from build123d import *

# Parameters (mm, degrees)
SKETCH1_W           = 914.4
SKETCH1_H           = 609.6
BOSS_EXTRUDE1_DEPTH = 6.35
SKETCH2_W           = 571.5
SKETCH2_H           = 266.7
CUT_EXTRUDE1_DEPTH  = 7.35
SKETCH3_W           = 101.6
SKETCH3_H           = 50.8
CUT_EXTRUDE2_DEPTH  = 7.35
FILLET1_R           = 12.7
SKETCH4_R           = 3.175
CUT_EXTRUDE3_DEPTH  = 7.35
SKETCH6_R           = 3.302
CUT_EXTRUDE5_DEPTH  = 6.35


with BuildPart() as part:
    # Sketch1 → Boss-Extrude1 (new body)
    with BuildSketch(Plane.ZY.offset(304.8)):
        with Locations((0, 304.8)):
            Rectangle(SKETCH1_W, SKETCH1_H)
    extrude(amount=BOSS_EXTRUDE1_DEPTH)

    # Sketch2 → Cut-Extrude1 (cut, through all)
    with BuildSketch(Plane.ZY.offset(311.15)):
        with Locations((0, 330.2)):
            Rectangle(SKETCH2_W, SKETCH2_H)
    extrude(amount=-CUT_EXTRUDE1_DEPTH, mode=Mode.SUBTRACT)

    # Sketch3 → Cut-Extrude2 (cut, through all)
    with BuildSketch(Plane.ZY.offset(311.15)):
        with Locations((-330.2, 69.85)):
            Rectangle(SKETCH3_W, SKETCH3_H)
        with Locations((330.2, 69.85)):
            Rectangle(SKETCH3_W, SKETCH3_H)
    extrude(amount=-CUT_EXTRUDE2_DEPTH, mode=Mode.SUBTRACT)

    # Fillet1
    fillet1_edges = [part.edges().sort_by_distance(p)[0] for p in [
        (-307.975, 196.85, -285.75),
        (-307.975, 463.55, -285.75),
        (-307.975, 463.55, 285.75),
        (-307.975, 196.85, 285.75),
        (-307.975, 44.45, -381),
        (-307.975, 95.25, -381),
        (-307.975, 95.25, -279.4),
        (-307.975, 44.45, -279.4),
        (-307.975, 95.25, 279.4),
        (-307.975, 95.25, 381),
        (-307.975, 44.45, 381),
        (-307.975, 44.45, 279.4),
    ]]
    fillet(fillet1_edges, radius=FILLET1_R)

    # Sketch4 → Cut-Extrude3 (cut, through all)
    with BuildSketch(Plane.ZY.offset(311.15)):
        with Locations((323.85, 244.475)):
            Circle(SKETCH4_R)
        with Locations((-323.85, 244.475)):
            Circle(SKETCH4_R)
        with Locations((-107.95, 158.75)):
            Circle(SKETCH4_R)
        with Locations((0, 158.75)):
            Circle(SKETCH4_R)
        with Locations((215.9, 158.75)):
            Circle(SKETCH4_R)
        with Locations((323.85, 158.75)):
            Circle(SKETCH4_R)
        with Locations((-323.85, 158.75)):
            Circle(SKETCH4_R)
        with Locations((-215.9, 158.75)):
            Circle(SKETCH4_R)
        with Locations((266.7, 31.75)):
            Circle(SKETCH4_R)
        with Locations((393.7, 31.75)):
            Circle(SKETCH4_R)
        with Locations((266.7, 107.95)):
            Circle(SKETCH4_R)
        with Locations((393.7, 107.95)):
            Circle(SKETCH4_R)
        with Locations((-266.7, 31.75)):
            Circle(SKETCH4_R)
        with Locations((-393.7, 31.75)):
            Circle(SKETCH4_R)
        with Locations((-393.7, 107.95)):
            Circle(SKETCH4_R)
        with Locations((-266.7, 107.95)):
            Circle(SKETCH4_R)
        with Locations((323.85, 330.2)):
            Circle(SKETCH4_R)
        with Locations((323.85, 415.925)):
            Circle(SKETCH4_R)
        with Locations((323.85, 501.65)):
            Circle(SKETCH4_R)
        with Locations((215.9, 501.65)):
            Circle(SKETCH4_R)
        with Locations((107.95, 501.65)):
            Circle(SKETCH4_R)
        with Locations((0, 501.65)):
            Circle(SKETCH4_R)
        with Locations((-107.95, 501.65)):
            Circle(SKETCH4_R)
        with Locations((-215.9, 501.65)):
            Circle(SKETCH4_R)
        with Locations((-323.85, 501.65)):
            Circle(SKETCH4_R)
        with Locations((-323.85, 415.925)):
            Circle(SKETCH4_R)
        with Locations((-323.85, 330.2)):
            Circle(SKETCH4_R)
    extrude(amount=-CUT_EXTRUDE3_DEPTH, mode=Mode.SUBTRACT)

    # Sketch6 → Cut-Extrude5 (cut)
    with BuildSketch(Plane.ZY.offset(311.15)):
        with Locations((431.8, 164.084)):
            Circle(SKETCH6_R)
        with Locations((431.8, 230.124)):
            Circle(SKETCH6_R)
        with Locations((431.8, 296.164)):
            Circle(SKETCH6_R)
        with Locations((431.8, 362.204)):
            Circle(SKETCH6_R)
        with Locations((431.8, 428.244)):
            Circle(SKETCH6_R)
        with Locations((431.8, 494.284)):
            Circle(SKETCH6_R)
        with Locations((-431.8, 230.124)):
            Circle(SKETCH6_R)
        with Locations((-431.8, 296.164)):
            Circle(SKETCH6_R)
        with Locations((-431.8, 362.204)):
            Circle(SKETCH6_R)
        with Locations((-431.8, 428.244)):
            Circle(SKETCH6_R)
        with Locations((-431.8, 494.284)):
            Circle(SKETCH6_R)
        with Locations((-431.8, 164.084)):
            Circle(SKETCH6_R)
    extrude(amount=-CUT_EXTRUDE5_DEPTH, mode=Mode.SUBTRACT)


solid = part.part
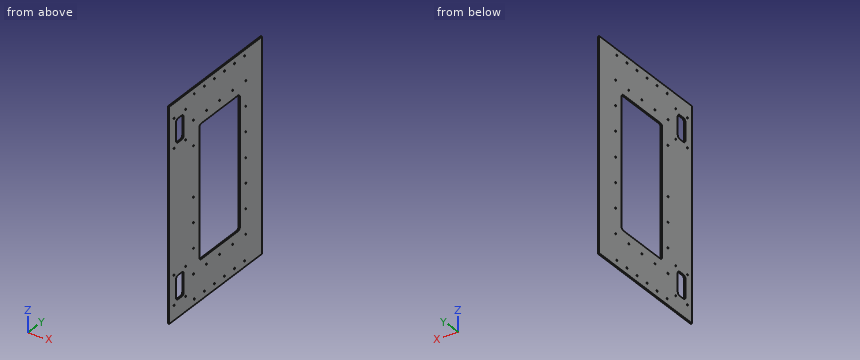
Model file for the job. Use its own axes, mm. Give positions to 0.01 mm unless a question says otherwise; leave off trailing zeros. Order: outer loops, then holes, each group sorted by start corner. A loop starts at its lowest first (then second) coordinate and runs counter-clockwise, first axis right, second up. Notation, with made-up numbers: (16, 59) -> (38, 59) arc R20 cw to (38, 81) -> close; hole circle Ø3 at (30.25, 13). An arc over 180 degrees is marked (long way). Use CSV: the item, a comma, the result in double quotes.
1. Band-saw the part on A-A, the plane z = 182. Give the cut face in (x, y).
Outcome:
outline,"(-311.15, 0) -> (-304.8, 0) -> (-304.8, 196.85) -> (-311.15, 196.85) -> close; (-311.15, 463.55) -> (-304.8, 463.55) -> (-304.8, 609.6) -> (-311.15, 609.6) -> close"
2. Drill centre lines: line 1 along Y through (x, z) = (-308.25, 215.9) (3 decimals); line 2 along Z through (x, y) = (-307.5, 301); line 3 along Y through (x, z) = (-310.5, 72.5). Where is each one in solid material? Low to high. Write a range as from..to.
Outcome:
line 1,"0..155.575, 161.925..196.85, 463.55..498.475, 504.825..609.6"
line 2,"-457.2..-285.75, 285.75..457.2"
line 3,"0..196.85, 463.55..609.6"
3. Band-saw the part on B-B, the plane x = -306. Count the separate pieces of the cut face and the enclosed holes in it, then the cut area to 3 significant figures.
Outcome:
separate pieces,"1"
enclosed holes,"42"
area,"394,000 mm²"
